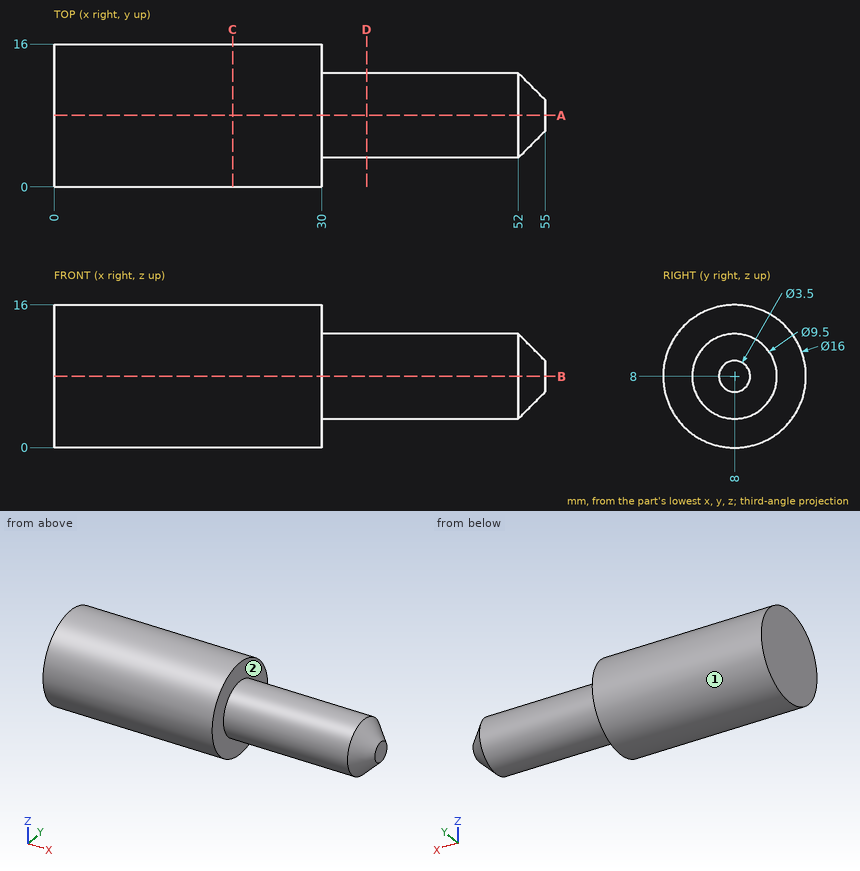
Geometry: see drawing. Coordinates: mm, zero at the bounding-box minimum. A direction names the side the tool comes from. Round coordinates to 2 decimals unless told otherwise and drop trailing zeros. Write each loop counter-clockwise with the first axis right and the second up, starting at its lowest first coordinate (ties: lowest second). Pieces come first, ordered by that corner, then holes. Notation, with made-up numbers: M -37,88 L -18,88 A32 ccw -18,118 Z; hole C -32.75,70.5 d9. An arc over 180 degrees is marked long. Answer in a Markdown table with one row per item. Add a question column.
(1) Ray query, L1, parallel to X at y = 8.75, z = 13.5; L2, parallel to Z at x = 52.5, y = 9; L3, parallel to Z at x = 14, y = 6.25. Return the intervals inside material, ascending.
(2) Cut plane C-C, the plane x = 20. Return the cut outline in (y, z), then the cut area to 3 significant figures.
(3) Reachability of the marked faces 1 and 2 from +Z, -Z, +X, -X, +Y, -Y: full face, straight path, thin tool, end or side. Return the list, or none.
(4) Cut plane D-D, the plane x = 35. Return the cut outline in (y, z), then the cut area to 3 significant figures.
(5) Contact query for flat-ended pins moving along their axis: pin 1 (8 mm diameter, centred on x = 8, y = 14, fed in from -Z); pin 2 (3 mm diameter, centred on y = 4.5, z = 7, fed in from +X); pin 3 (6 mm diameter, centred on x = 38, z = 2, fed in from +Y). Output: stop coordinate, or through.
(6) Cut plane A-A, the plane y = 8. Return the cut outline in (x, z), then the cut area to 4 significant figures.
Established:
| question | item | result |
|---|---|---|
| 1 | L1 | 0 to 30 |
| 1 | L2 | 3.87 to 12.13 |
| 1 | L3 | 0.19 to 15.81 |
| 2 | outline | C 8,8 d16 |
| 2 | area | 201 mm² |
| 3 | face 1 | +X, -X |
| 3 | face 2 | +X |
| 4 | outline | C 8,8 d9.5 |
| 4 | area | 70.9 mm² |
| 5 | pin 1 | z = 0.25 |
| 5 | pin 2 | x = 54.61 |
| 5 | pin 3 | y = 11.68 |
| 6 | outline | M 0,0 L 30,0 L 30,3.25 L 52,3.25 L 55,6.25 L 55,9.75 L 52,12.75 L 30,12.75 L 30,16 L 0,16 Z |
| 6 | area | 708.5 mm² |
